Design review of the part built by this model. Coordinates are the model's own, in mm. A direction names the side the tool comes from. Coordinates: 2 decimals unless noted, no trailing zeros. Write each loop counter-clockwise with the first axis right and the second up, starting at its lowest first coordinate (ties: lowest second). Pieces come first, ordered by that corner, then holes. Notation, with made-up numbers: M -1.5,38.5 L 15.5,38.5 A18 cw 15.5,49.5 Z; hole C 41,-22.75 d10. An arc over 180 degrees is marked long. Write item = value, one per line.
```python
from build123d import *

# Parameters (mm, degrees)
SKETCH1_W      = 136.944523068
SKETCH1_H      = 30
SKETCH1_W_2    = 7.9375
SKETCH1_H_2    = 6.35
EXTRUDE1_DEPTH = 3.175


with BuildPart() as part:
    # Sketch1 → Extrude1 (new body)
    with BuildSketch(Plane(origin=(0, 0, 0), x_dir=(1, 0, 0), z_dir=(0, 1, 0))):
        Polygon((-67.158636898, 70.484310302), (-67.158636898, 74.492800404), (-68.408636898, 74.492800404), (-68.408636898, 76.742800404), (-67.158636898, 76.742800404), (-67.158636898, 85.234310302), (-82.88813161, 85.234310302), (-82.88813161, 91.584310302), (-92.88813161, 91.584310302), (-92.88813161, -10.015689698), (-82.88813161, -10.015689698), (-82.88813161, -3.665689698), (-67.158636898, -3.665689698), (-67.158636898, 4.825820201), (-68.408636898, 4.825820201), (-68.408636898, 7.075820201), (-67.158636898, 7.075820201), (-67.158636898, 11.084310302), (-64.258636898, 11.084310302), (-64.258636898, 7.075820201), (-63.008636898, 7.075820201), (-63.008636898, 4.825820201), (-64.258636898, 4.825820201), (-64.258636898, -3.665689698), (2.20186839, -3.665689698), (2.20186839, -10.015689698), (12.20186839, -10.015689698), (12.20186839, -3.665689698), (18.744143558, -3.665689698), (18.744143558, 5.171032224), (17.494143558, 5.171032224), (17.494143558, 7.421032224), (18.744143558, 7.421032224), (18.744143558, 11.084310302), (21.644143558, 11.084310302), (21.644143558, 7.421032224), (22.894143558, 7.421032224), (22.894143558, 5.171032224), (21.644143558, 5.171032224), (21.644143558, -3.665689698), (74.914143558, -3.665689698), (74.914143558, -10.015689698), (84.914143558, -10.015689698), (84.914143558, 91.584310302), (74.914143558, 91.584310302), (74.914143558, 85.234310302), (21.644143558, 85.234310302), (21.644143558, 76.397588381), (22.894143558, 76.397588381), (22.894143558, 74.147588381), (21.644143558, 74.147588381), (21.644143558, 70.484310302), (18.744143558, 70.484310302), (18.744143558, 74.147588381), (17.494143558, 74.147588381), (17.494143558, 76.397588381), (18.744143558, 76.397588381), (18.744143558, 85.234310302), (12.20186839, 85.234310302), (12.20186839, 91.584310302), (2.20186839, 91.584310302), (2.20186839, 85.234310302), (-64.258636898, 85.234310302), (-64.258636898, 76.742800404), (-63.008636898, 76.742800404), (-63.008636898, 74.492800404), (-64.258636898, 74.492800404), (-64.258636898, 70.484310302), align=None)
        with Locations((-4.072635431, 40.784310302)):
            Rectangle(SKETCH1_W, SKETCH1_H, mode=Mode.SUBTRACT)
        with Locations((73.709900913, 40.784310302)):
            Rectangle(SKETCH1_W_2, SKETCH1_H_2, mode=Mode.SUBTRACT)
    extrude(amount=EXTRUDE1_DEPTH)


solid = part.part
```
Q1. The part is to be moulded in two halves that separate along X. For faces 4 (the flat face through (21.644, 2, -9)), 5 (the flat face through (-5, 0, -19)), 6 (the flat face through (-92.888, 2, -41)), say which applies: +X half, -X half, draft (parallel to the pull), parting line (faces both ways), or undercut.
Check result:
face_4 = undercut
face_5 = draft
face_6 = -X half
Q2. Consider section B-B, the plane z = -79.5. State the section outline as (x, y) points (3 decimals), and give its area (3 significant figures).
Check result:
outline = M -92.888,0 L -67.159,0 L -67.159,3.175 L -92.888,3.175 Z; M -64.259,0 L 18.744,0 L 18.744,3.175 L -64.259,3.175 Z; M 21.644,0 L 84.914,0 L 84.914,3.175 L 21.644,3.175 Z
area = 546 mm²
Q3. Wall thickness on line 1 (X direction, y = 2.55, z = 5); line 2 (X direction, y = 0.4, z = -43.5); line 3 (Z direction, x = -20, y = 2.9): over which ranges is each line inside the solid? List them lowest first.
Check result:
line_1 = -92.89 to -82.89, 2.2 to 12.2, 74.91 to 84.91
line_2 = -92.89 to -72.54, 64.4 to 69.74, 77.68 to 84.91
line_3 = -85.23 to -55.78, -25.78 to 3.67
Q4. Consider section C-C, the plane z = -35. State the section outline as (x, y) points (3 decimals).
Check result:
outline = M -92.888,0 L -72.545,0 L -72.545,3.175 L -92.888,3.175 Z; M 64.4,0 L 84.914,0 L 84.914,3.175 L 64.4,3.175 Z
Q5. Machinability: for faces 1 (the flat face through (-31, 2, -85.234)), 2 (the flat face through (77.679, 2, -41)), 3 (the flat face through (2.202, 2, 7)), which of the approach directions +Z, -Z, +X, -X, +Y, -Y give a long, thin tool a straight path to every point of the face, cutting with its end or side? Answer none if there is none.
Check result:
face_1 = -Z, +Y, -Y
face_2 = +Y, -Y
face_3 = +Z, +Y, -Y
Q6. Consider section A-A, the plane x = -20. State the section outline as (y, z) points (3 decimals), and give its area (3 significant figures).
Check result:
outline = M 0,-85.234 L 3.175,-85.234 L 3.175,-55.784 L 0,-55.784 Z; M 0,-25.784 L 3.175,-25.784 L 3.175,3.666 L 0,3.666 Z
area = 187 mm²
Q7. For P1, Ø1.4, axis at x = 18, y = 2, coming from the -Z side; P2, Ø1.4, axis at x = 22.5, y = 1.5, coming from the +Z side, all flat-tipped, find the tip position at first contact; note any pin that passes through.
Check result:
P1 = -85.23
P2 = 3.67
Q8. Consider section D-D, the plane x = 67.5. State the section outline as (y, z) points (3 decimals).
Check result:
outline = M 0,-85.234 L 3.175,-85.234 L 3.175,3.666 L 0,3.666 Z
